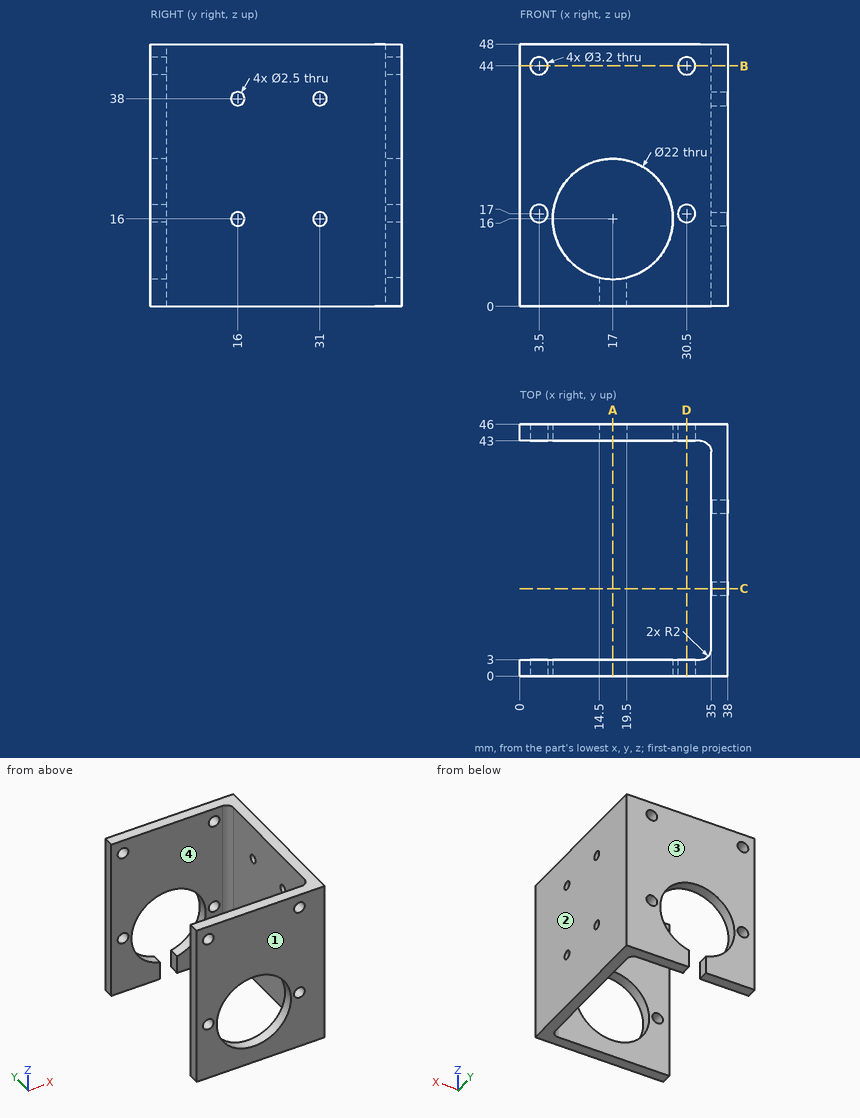
Verification items for this drawing (mm, ordinates from the low corner). Coordinates: 2 decimals unless noted, no trailing zeros. Order: outer loops, then holes, each group sorted by start corner. A loop starts at its lowest first (then second) coordinate and runs counter-clockwise, first axis right, second up.
Q1. Sectioned sample at C-C on y = 16. Record the cut outline in (x, z).
Reply:
outline: (35, 0) - (38, 0) - (38, 14.75) - (35, 14.75) - close; (35, 17.25) - (38, 17.25) - (38, 36.75) - (35, 36.75) - close; (35, 39.25) - (38, 39.25) - (38, 48) - (35, 48) - close
Q2. Depth check by flat-ended pin: pin 1 Ø3.5 at (x, z) = (3.5, 17) entering from +Y; pin 2 Ø1.9 at (x, z) = (30.5, 17) entering from -Y; pin 3 Ø8 at (y, z) = (35, 40) entering from -X. Enter the tip coordinate at first touch or a pass-through.
Reply:
pin 1: stops at y = 46
pin 2: passes through
pin 3: stops at x = 35
Q3. Thickness scan on probe 1 along Z at (x, y) = (36.9, 16); probe 2 along Z at (x, y) = (30.5, 1.15); probe 3 along Y at (x, z) = (33, 26). Record the ranges inside material, lowest first.
Reply:
probe 1: z = 0 to 14.75, 17.25 to 36.75, 39.25 to 48
probe 2: z = 0 to 15.4, 18.6 to 42.4, 45.6 to 48
probe 3: y = 0 to 3, 43 to 46
Q4. Sectioned sample at B-B on z = 44. Record the cut outline in (x, y), and give its area (3 significant figures).
Reply:
outline: (0, 0) - (1.9, 0) - (1.9, 3) - (0, 3) - close; (0, 43) - (1.9, 43) - (1.9, 46) - (0, 46) - close; (5.1, 0) - (28.9, 0) - (28.9, 3) - (5.1, 3) - close; (5.1, 43) - (28.9, 43) - (28.9, 46) - (5.1, 46) - close; (32.1, 0) - (38, 0) - (38, 46) - (32.1, 46) - (32.1, 43) - (33, 43) arc R2 cw to (35, 41) - (35, 5) arc R2 cw to (33, 3) - (32.1, 3) - close
area: 311 mm2
Q5. Sectioned sample at A-A on x = 17. Record the cut outline in (y, z), and give its area (3 significant figures).
Reply:
outline: (0, 0) - (3, 0) - (3, 5) - (0, 5) - close; (0, 27) - (3, 27) - (3, 48) - (0, 48) - close; (43, 27) - (46, 27) - (46, 48) - (43, 48) - close
area: 141 mm2
Q6. Draft check along Y on the marked faces 1, 2, 3 and 4. Enter one of: released by +Y, released by -Y, zero draft, split by the parting line, or undercut.
Reply:
face 1: released by -Y
face 2: zero draft
face 3: released by +Y
face 4: undercut
Q7. Sectioned sample at D-D on x = 30.5. Record the cut outline in (y, z), and give its area (3 significant figures).
Reply:
outline: (0, 0) - (3, 0) - (3, 15.4) - (0, 15.4) - close; (0, 18.6) - (3, 18.6) - (3, 42.4) - (0, 42.4) - close; (0, 45.6) - (3, 45.6) - (3, 48) - (0, 48) - close; (43, 0) - (46, 0) - (46, 15.4) - (43, 15.4) - close; (43, 18.6) - (46, 18.6) - (46, 42.4) - (43, 42.4) - close; (43, 45.6) - (46, 45.6) - (46, 48) - (43, 48) - close
area: 250 mm2
